Verification items for the finished model (mm, model axes). Face numbers are marked on the shaded views. A direction names the side the tool comes from. Round coordinates to 2 decimals unless told otherwise and drop trailing zeros. Order: outer loops, then holes, each group sorted by start corner. A loop starts at its lowest first (then second) coordinate and runs counter-clockwise, first axis right, second up. Notation, with made-up numbers: (37.5, 13.25) -> (51.5, 13.25) arc R21 ccw to (51.5, 41.25) -> close; hole circle Ø4 at (28, 5.5). An arc over 180 degrees is marked (long way). Put each result on its own line as item: value.
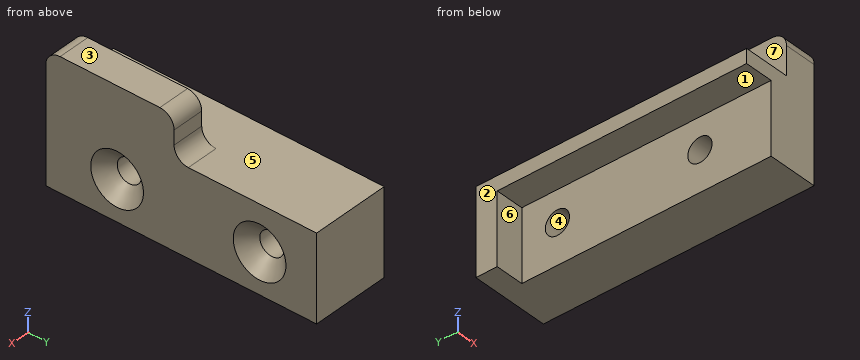
```python
from build123d import *

# Parameters (mm, degrees)
PAD009_DEPTH    = 35
SKETCH016_R     = 1.7
POCKET005_DEPTH = 11.001
CHAMFER_SIZE    = 2
SKETCH017_W     = 12
SKETCH017_H     = 3
PAD010_DEPTH    = 11
SKETCH019_W     = 6
SKETCH019_H     = 18
PAD011_DEPTH    = 4.5
FILLET_R        = 2


with BuildPart() as part:
    # Sketch015 → Pad009 (new body)
    with BuildSketch(Plane.XZ):
        Polygon((-4, 0), (0, 0), (0, -10), (7, -10), (7, 2), (-4, 2), align=None)
    extrude(amount=PAD009_DEPTH)

    # Sketch016 (on Face4 of Pad009) → Pocket005 (cut, through all)
    with BuildSketch(Plane(origin=(7, 0, 0), x_dir=(0, 0, 1), z_dir=(1, 0, 0))):
        with Locations((-4.354385, 25)):
            Circle(SKETCH016_R)
        with Locations((-4.354385, 5)):
            Circle(SKETCH016_R)
    extrude(amount=-POCKET005_DEPTH, mode=Mode.SUBTRACT)

    # Chamfer
    chamfer_edges = [part.edges().sort_by_distance(p)[0] for p in [
        (7, -25, -6.054385),
        (7, -5, -6.054385),
    ]]
    chamfer(chamfer_edges, length=CHAMFER_SIZE)

    # Sketch017 (on Face4 of Chamfer) → Pad010 (join)
    with BuildSketch(Plane(origin=(7, 0, 0), x_dir=(0, 0, 1), z_dir=(1, 0, 0))):
        with Locations((-4, -1.5)):
            Rectangle(SKETCH017_W, SKETCH017_H)
    extrude(amount=-PAD010_DEPTH)

    # Sketch019 (on Face4 of Pad010) → Pad011 (join)
    with BuildSketch(Plane(origin=(7, 0, 0), x_dir=(0, 0, 1), z_dir=(1, 0, 0))):
        with Locations((5, 26)):
            Rectangle(SKETCH019_W, SKETCH019_H)
    extrude(amount=-PAD011_DEPTH)

    # Fillet
    fillet_edges = [part.edges().sort_by_distance(p)[0] for p in [
        (4.75, -17, 2),
        (4.75, -17, 8),
        (4.75, -35, 8),
    ]]
    fillet(fillet_edges, radius=FILLET_R)


solid = part.part
```
Item 1: Material ranges on line 1 along Z through (x, y) = (1.3, -5); line 2 along X through (y, z) = (-30, -5.75); line 3 along Y through (x, z) = (-2.75, -6.25), recorded low to high.
Geometry check:
line 1: -10 to -6.05, -2.65 to 2
line 2: 0 to 7
line 3: 0 to 3
Item 2: Sectioned sample at A-A, the plane y = -25. Record the boundary of the cut face in (x, z).
Geometry check:
outline: (-4, 0) -> (0, 0) -> (0, -2.65) -> (5, -2.65) -> (7, -0.65) -> (7, 8) -> (2.5, 8) -> (2.5, 2) -> (-4, 2) -> close; (0, -10) -> (7, -10) -> (7, -8.05) -> (5, -6.05) -> (0, -6.05) -> close
Item 3: Depth check by flat-ended pin: pin 1 Ø1 at (x, y) = (0.5, -10.5) entering from +Z; pin 2 Ø6.5 at (y, z) = (-24, 5.5) entering from -X; pin 3 Ø2 at (x, z) = (-3, -4.5) entering from -Y. Enter the tip coordinate at first touch or a pass-through.
Geometry check:
pin 1: z = 2
pin 2: x = 2.5
pin 3: y = 0
Item 4: Release check for a two-part mould opening along Z. For the marked faces 1, 2, 3 and 4 record: pulls with the +Z half, pulls with the -Z half, needs draft (parallel to the pull), parting line crosses it, or undercut.
Geometry check:
face 1: pulls with the -Z half
face 2: needs draft
face 3: pulls with the +Z half
face 4: undercut
Item 5: Tool access check on the marked faces 5, 6 and 7. Record the directions out of +Z, -Z, +X, -X, +Y, -Y that give a thin tool (end or side, any length) a straight path to the whole face; none if there is none.
Geometry check:
face 5: +Z, -X, +Y
face 6: -Z, -X, -Y
face 7: +Z, -X, +Y, -Y
Item 6: Sectioned sample at C-C, the plane y = -5. Record the boundary of the cut face in (x, z), then the cut area to 3 significant figures.
Geometry check:
outline: (-4, 0) -> (0, 0) -> (0, -2.65) -> (5, -2.65) -> (7, -0.65) -> (7, 2) -> (-4, 2) -> close; (0, -10) -> (7, -10) -> (7, -8.05) -> (5, -6.05) -> (0, -6.05) -> close
area: 64.2 mm2
Item 7: Sectioned sample at B-B, the plane x = 4. Record the boundary of the cut face in (y, z).
Geometry check:
outline: (-35, -10) -> (3, -10) -> (3, 2) -> (-15, 2) arc R2 cw to (-17, 4) -> (-17, 6) arc R2 ccw to (-19, 8) -> (-33, 8) arc R2 ccw to (-35, 6) -> close; hole circle Ø3.4 at (-25, -4.35); hole circle Ø3.4 at (-5, -4.35)
Item 8: Sectioned sample at D-D, the plane y = -32. Record the boundary of the cut face in (x, z), then the cut area to 3 significant figures.
Geometry check:
outline: (-4, 0) -> (0, 0) -> (0, -10) -> (7, -10) -> (7, 8) -> (2.5, 8) -> (2.5, 2) -> (-4, 2) -> close
area: 119 mm2
